Can you work these out from the model? Positions are in its coordinate system, mm. Face numbers are marked on the shaded views. A direction names the side the tool comes from. Give positions to 0.01 mm unless a question says otherwise; leave off trailing zeros. Order: outer loops, then holes, each group sorted by start corner. A loop starts at its lowest first (then second) coordinate and runs counter-clockwise, first axis right, second up. Notation, with made-up numbers: (5, -4.5) -> (45, -4.5) arc R21 cw to (45, 12.5) -> close; hole circle Ø7 at (-29, 51). An arc over 180 degrees is marked (long way). Answer as a JSON object with one key per item and string values.
```python
from build123d import *

# Parameters (mm, degrees)
SKETCH_1_R          = 4.5
SKETCH_1_R_2        = 2.6
EXTRUDE_1_DEPTH     = 2.8
SKETCH_2_R          = 0.75
SKETCH_2_R_2        = 2.6
EXTRUDE_4_DEPTH     = 2.5
CUT_EXTRUDE_START   = -1
SKETCH_4_R          = 3.85
SKETCH_4_R_2        = 3.35
SKETCH_4_R_3        = 3.1
SKETCH_4_R_4        = 2.6
CUT_EXTRUDE_1_DEPTH = 1


with BuildPart() as part:
    # 草图1 → 凸台-拉伸1 (new body)
    with BuildSketch(Plane(origin=(0, 0, 0), x_dir=(1, 0, 0), z_dir=(0, 1, 0))):
        with Locations(Location((0, 0, 0), (0, 0, 270))):
            Circle(SKETCH_1_R)
        with Locations(Location((0, 0, 0), (0, 0, 270))):
            Circle(SKETCH_1_R_2, mode=Mode.SUBTRACT)
    extrude(amount=EXTRUDE_1_DEPTH)

    # 草图2 → 凸台-拉伸4 (add)
    with BuildSketch(Plane(origin=(0, 2.8, 0), x_dir=(1, 0, 0), z_dir=(0, 1, 0))):
        with BuildLine():
            Line((-17.34846223, 1.606822932), (-8.172576507, 3.533758933))
            ThreePointArc((-8.172576507, 3.533758933), (-5.163039226, 5.163039226), (-3.533758933, 8.172576507))
            Line((-3.533758933, 8.172576507), (-1.606822932, 17.34846223))
            ThreePointArc((-1.606822932, 17.34846223), (-1.258440316, 17.919320303), (-0.628169435, 18.142944996))
            Line((-0.628169435, 18.142944996), (0.628169435, 18.142944996))
            ThreePointArc((0.628169435, 18.142944996), (1.258440316, 17.919320303), (1.606822932, 17.34846223))
            Line((1.606822932, 17.34846223), (3.533758933, 8.172576507))
            ThreePointArc((3.533758933, 8.172576507), (5.163039226, 5.163039226), (8.172576507, 3.533758933))
            Line((8.172576507, 3.533758933), (17.34846223, 1.606822932))
            ThreePointArc((17.34846223, 1.606822932), (17.919320303, 1.258440316), (18.142944996, 0.628169435))
            Line((18.142944996, 0.628169435), (18.142944996, -0.628169435))
            ThreePointArc((18.142944996, -0.628169435), (17.919320303, -1.258440316), (17.34846223, -1.606822932))
            Line((17.34846223, -1.606822932), (8.172576507, -3.533758933))
            ThreePointArc((8.172576507, -3.533758933), (5.163039226, -5.163039226), (3.533758933, -8.172576507))
            Line((3.533758933, -8.172576507), (1.606822932, -17.34846223))
            ThreePointArc((1.606822932, -17.34846223), (1.258440316, -17.919320303), (0.628169435, -18.142944996))
            Line((0.628169435, -18.142944996), (-0.628169435, -18.142944996))
            ThreePointArc((-0.628169435, -18.142944996), (-1.258440316, -17.919320303), (-1.606822932, -17.34846223))
            Line((-1.606822932, -17.34846223), (-3.533758933, -8.172576507))
            ThreePointArc((-3.533758933, -8.172576507), (-5.163039226, -5.163039226), (-8.172576507, -3.533758933))
            Line((-8.172576507, -3.533758933), (-17.34846223, -1.606822932))
            ThreePointArc((-17.34846223, -1.606822932), (-17.919320303, -1.258440316), (-18.142944996, -0.628169435))
            Line((-18.142944996, -0.628169435), (-18.142944996, 0.628169435))
            ThreePointArc((-18.142944996, 0.628169435), (-17.919320303, 1.258440316), (-17.34846223, 1.606822932))
        make_face()
        with Locations(Location((-7, 0, 0), (0, 0, 270))):
            Circle(SKETCH_2_R, mode=Mode.SUBTRACT)
        with Locations(Location((-10, 0, 0), (0, 0, 270))):
            Circle(SKETCH_2_R, mode=Mode.SUBTRACT)
        with Locations(Location((-13, 0, 0), (0, 0, 270))):
            Circle(SKETCH_2_R, mode=Mode.SUBTRACT)
        with Locations(Location((-16, 0, 0), (0, 0, 270))):
            Circle(SKETCH_2_R, mode=Mode.SUBTRACT)
        with Locations(Location((0, 7, 0), (0, 0, 270))):
            Circle(SKETCH_2_R, mode=Mode.SUBTRACT)
        with Locations(Location((0, 10, 0), (0, 0, 270))):
            Circle(SKETCH_2_R, mode=Mode.SUBTRACT)
        with Locations(Location((0, 13, 0), (0, 0, 270))):
            Circle(SKETCH_2_R, mode=Mode.SUBTRACT)
        with Locations(Location((0, 16, 0), (0, 0, 270))):
            Circle(SKETCH_2_R, mode=Mode.SUBTRACT)
        with Locations(Location((7, 0, 0), (0, 0, 270))):
            Circle(SKETCH_2_R, mode=Mode.SUBTRACT)
        with Locations(Location((10, 0, 0), (0, 0, 270))):
            Circle(SKETCH_2_R, mode=Mode.SUBTRACT)
        with Locations(Location((13, 0, 0), (0, 0, 270))):
            Circle(SKETCH_2_R, mode=Mode.SUBTRACT)
        with Locations(Location((16, 0, 0), (0, 0, 270))):
            Circle(SKETCH_2_R, mode=Mode.SUBTRACT)
        with Locations(Location((0, -7, 0), (0, 0, 270))):
            Circle(SKETCH_2_R, mode=Mode.SUBTRACT)
        with Locations(Location((0, -10, 0), (0, 0, 270))):
            Circle(SKETCH_2_R, mode=Mode.SUBTRACT)
        with Locations(Location((0, -13, 0), (0, 0, 270))):
            Circle(SKETCH_2_R, mode=Mode.SUBTRACT)
        with Locations(Location((0, -16, 0), (0, 0, 270))):
            Circle(SKETCH_2_R, mode=Mode.SUBTRACT)
        with Locations(Location((0, 0, 0), (0, 0, 270))):
            Circle(SKETCH_2_R_2, mode=Mode.SUBTRACT)
    extrude(amount=EXTRUDE_4_DEPTH)

    # 草图4 → 切除-拉伸1 (cut)
    # profile 1 of 2: a face of its own
    with BuildSketch(Plane(origin=(0, 5.3, 0), x_dir=(1, 0, 0), z_dir=(0, 1, 0)).offset(CUT_EXTRUDE_START)):
        with Locations(Location((0, 0, 0), (0, 0, 270))):
            Circle(SKETCH_4_R)
        with Locations(Location((0, 0, 0), (0, 0, 270))):
            Circle(SKETCH_4_R_2, mode=Mode.SUBTRACT)
    # profile 2 of 2: a face of its own
    with BuildSketch(Plane(origin=(0, 5.3, 0), x_dir=(1, 0, 0), z_dir=(0, 1, 0)).offset(CUT_EXTRUDE_START)):
        with Locations(Location((0, 0, 0), (0, 0, 270))):
            Circle(SKETCH_4_R_3)
        with Locations(Location((0, 0, 0), (0, 0, 270))):
            Circle(SKETCH_4_R_4, mode=Mode.SUBTRACT)
    extrude(amount=CUT_EXTRUDE_1_DEPTH, mode=Mode.SUBTRACT)


solid = part.part
```
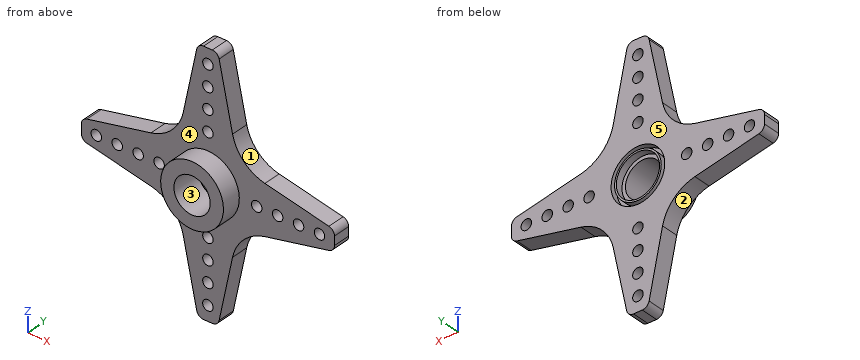
1. Please list where these lines run through material, in increasing order: L1, parallel to Y at x = -13.5, z = 1; L2, parallel to X at y = 4.6, z = -16; L3, parallel to Z at x = 12.5, y = 3.2 (3 decimals).
Worked answers:
{"L1": "2.8 to 5.3", "L2": "-1.89 to -0.75, 0.75 to 1.89", "L3": "-2.625 to -0.559, 0.559 to 2.625"}
2. If we section it at D-D on z = 0: Count the separate pieces of the cut face and the enclosed holes in it, then the cut area to 3 significant figures.
Worked answers:
{"separate pieces": "10", "enclosed holes": "0", "area": "56.4 mm²"}
3. Will these pins go through, and if not, where does the flat tip stop? pin 1 Ø18 at (x, z) = (0.5, 2.5) entering from -Y; pin 2 Ø1.5 at (x, z) = (10.5, 2) entering from -Y; pin 3 Ø1.4 at (x, z) = (16, 0) entering from +Y; pin 4 Ø2.5 at (x, z) = (-1.5, -1) entering from +Y.
Worked answers:
{"pin 1": "y = 0", "pin 2": "y = 2.8", "pin 3": "through", "pin 4": "y = 4.3"}
4. If we section it at C-C on y = 0.9: Please give me the cut outline in (x, z), then the cut area to 3 significant figures.
Worked answers:
{"outline": "circle Ø9 at (0, 0); hole circle Ø5.2 at (0, 0)", "area": "42.4 mm²"}
5. For the marked faces 4 and 5, which set-ups out of +Z, -Z, +X, -X, +Y, -Y let a thin tool reach every point of the face, with its end or its side?
Worked answers:
{"face 4": "-Y", "face 5": "+Z, -Z, +X, -X, +Y"}
6. If we mould it in two halves opening along Z, with no side actions, what happens to the marked faces 1, 2 and 3? For each: +Z half, -Z half, draft (parallel to the pull), parting line (faces both ways), or undercut.
Worked answers:
{"face 1": "+Z half", "face 2": "-Z half", "face 3": "undercut"}
7. If we section it at A-A on x = -16: Please give me the cut outline in (y, z), then the cut area to 3 significant figures.
Worked answers:
{"outline": "(2.8, -1.89) -> (5.3, -1.89) -> (5.3, -0.75) -> (2.8, -0.75) -> close; (2.8, 0.75) -> (5.3, 0.75) -> (5.3, 1.89) -> (2.8, 1.89) -> close", "area": "5.70 mm²"}
8. If we section it at B-B on z = -10: Please give me the cut outline in (x, y), then the cut area to 3 significant figures.
Worked answers:
{"outline": "(-3.15, 2.8) -> (-0.75, 2.8) -> (-0.75, 5.3) -> (-3.15, 5.3) -> close; (0.75, 2.8) -> (3.15, 2.8) -> (3.15, 5.3) -> (0.75, 5.3) -> close", "area": "12.0 mm²"}
